Source: three-view drawing plus pictorial views. Frame: mm from the lowest corner of the part. Give positions to 0.01 mm unless a question says otherwise; leave off trailing zeros. Loops run counter-clockwise (first coordinate to the right, second up) from the corner with the lowest first, then second, coordinate; pieces in that order, holes last. Notation, with made-up numbers: (34.25, -5.5) -> (47.25, -5.5) arc R7 cw to (47.25, 0.5) -> close; hole circle Ø1 at (12, 18.5). An arc over 180 degrees is marked (long way). Answer in a Markdown table with one row per item. Add a question column.
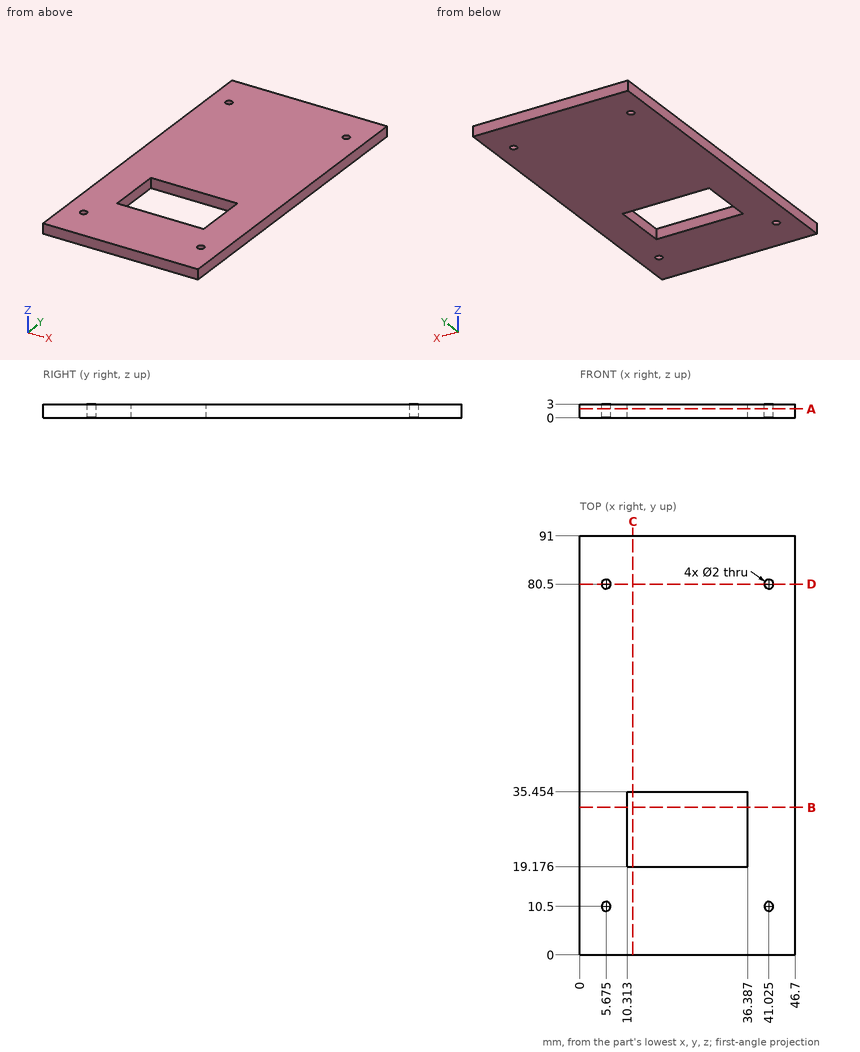
(1) Material intervals for line 1 along X through (y, z) = (80.5, 2.2) (1 decimal); line 2 along X through (y, z) = (28, 1.45); line 3 along Y through (x, z) = (27, 1.7), sorted ascending. Write a range as from..to.
(2) Cut plane A-A on z = 1.95. Return the cut outline in (x, y) (1 decimal).
(3) Cut plane C-C on x = 11.5. Return the cut outline in (y, z).
(4) Pin query (flat end, axial travel): pin 1 Ø1.6 at (x, y) = (5.675, 10.5) entering from +Z. Return the tip coordinate at first contact, or that it passes through.
(5) Cut plane B-B on y = 32. Return the cut outline in (x, z).
(6) Cut plane D-D on y = 80.5. Return the cut outline in (x, z) (1 decimal), then the cut area to 3 significant figures.
Answer list:
| question | item | result |
|---|---|---|
| 1 | line 1 | x = 0..4.7, 6.7..40, 42..46.7 |
| 1 | line 2 | x = 0..10.31, 36.39..46.7 |
| 1 | line 3 | y = 0..19.18, 35.45..91 |
| 2 | outline | (0, 0) -> (46.7, 0) -> (46.7, 91) -> (0, 91) -> close; hole circle Ø2 at (5.7, 10.5); hole circle Ø2 at (5.7, 80.5); hole (10.3, 19.2) -> (36.4, 19.2) -> (36.4, 35.5) -> (10.3, 35.5) -> close; hole circle Ø2 at (41, 10.5); hole circle Ø2 at (41, 80.5) |
| 3 | outline | (0, 0) -> (19.18, 0) -> (19.18, 3) -> (0, 3) -> close; (35.45, 0) -> (91, 0) -> (91, 3) -> (35.45, 3) -> close |
| 4 | pin 1 | passes through |
| 5 | outline | (0, 0) -> (10.31, 0) -> (10.31, 3) -> (0, 3) -> close; (36.39, 0) -> (46.7, 0) -> (46.7, 3) -> (36.39, 3) -> close |
| 6 | outline | (0, 0) -> (4.7, 0) -> (4.7, 3) -> (0, 3) -> close; (6.7, 0) -> (40, 0) -> (40, 3) -> (6.7, 3) -> close; (42, 0) -> (46.7, 0) -> (46.7, 3) -> (42, 3) -> close |
| 6 | area | 128 mm² |
